Build history of the part. All positions in model axes, mm. Face numbers are marked on the shaded views. A direction names the side the tool comes from. Give positions to 0.01 mm unless a question says otherwise; leave off trailing zeros. Loops run counter-clockwise (first coordinate to the right, second up) from the corner with the lowest first, then second, coordinate; pieces in that order, holes last. Notation, with made-up numbers: (5, 16) -> (18, 16) arc R24 cw to (18, 39) -> close; hole circle Ø5 at (-36, 16.25). An arc over 180 degrees is marked (long way). Answer as a JSON object with one key per item and string values. Group by question number.
Q1. Two-plate mould, pull along X, no slides. Class the marked faces 3, 4 and 5: pulls with the +X half, pulls with the -X half, needs draft (parallel to the pull), parting line crosses it, or undercut.
Q2. Band-saw the part on B-B, the plane y = 1. Write the cut outline in (x, z), plus the area to 3 significant figures.
Q3. Drop flat-ended pins along their axis: pin 1 (1 mm diameter, centred on x = -6.5, y = 8, fed in from -Z); pin 2 (5 mm diameter, centred on x = -2.5, z = 5.5, fed in from +Y); pin 3 (3 mm diameter, centred on x = 5.5, z = 1, fed in from +Y). Give the stop position or say it passes through.
Q4. Band-saw the part on A-A, the plane z = 8. Write the cut outline in (x, y).
Q5. Wall check: probe 1 along X at (y, z) = (2.3, 0); probe 2 along Z at (x, y) = (0, 1.2). Give the ranges that are in metal, low to high. Write a range as from..to.
Q6. Tool access for the marked faces 1 and 2: list every direction of +Z, -Z, +X, -X, +Y, -Y with a clear straight run to the whole face (end or side of a thin tool).
from build123d import *

# Parameters (mm, degrees)
SKETCH4_R          = 4.7752
CUT_EXTRUDE1_DEPTH = 12.446
FILLET2_R          = 5.08


with BuildPart() as part:
    # Sketch3 → Revolve3 (revolve)
    with BuildSketch(Plane.XY):
        Polygon((7.1628, 1.8288), (7.1628, 5.1054), (0, 5.1054), (0, 0), (9.398, 0), (9.398, 1.8288), align=None)
        with BuildLine():
            ThreePointArc((0, 5.1054), (5.231120596, 6.316339666), (9.398, 9.7028))
            Line((9.398, 9.7028), (9.398, 5.1054))
            Line((9.398, 5.1054), (7.1628, 5.1054))
            Line((7.1628, 5.1054), (0, 5.1054))
        make_face()
    revolve(axis=Axis((0, 0, 0), (0, 1, 0)))

    # Sketch4 → Cut-Extrude1 (cut)
    with BuildSketch(Plane.XZ):
        Circle(SKETCH4_R)
    extrude(amount=-CUT_EXTRUDE1_DEPTH, mode=Mode.SUBTRACT)

    # Fillet2
    fillet2_edges = [part.edges().sort_by_distance(p)[0] for p in [
        (-4.7752, 6.105113597, 2e-09),
    ]]
    fillet(fillet2_edges, radius=FILLET2_R)


solid = part.part
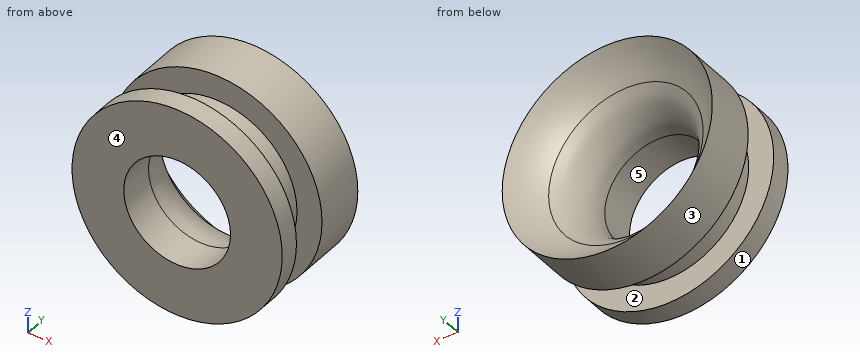
Worked answers:
{
 "1": {"face 3": "parting line crosses it", "face 4": "needs draft", "face 5": "undercut"},
 "2": {"outline": "circle Ø18.8 at (0, 0); hole circle Ø9.55 at (0, 0)", "area": "206 mm2"},
 "3": {"pin 1": "z = -7.23", "pin 2": "y = 8.72", "pin 3": "y = 7.45"},
 "4": {"outline": "(-4.93, 0) -> (4.93, 0) -> (4.93, 1.83) -> (-4.93, 1.83) -> close; (-4.93, 5.11) -> (4.93, 5.11) -> (4.93, 9.7) arc R8.82 cw to (-4.93, 9.7) -> close"},
 "5": {"probe 1": "-7.16..-4.78, 4.78..7.16", "probe 2": "-9.4..-4.78, 4.78..9.4"},
 "6": {"face 1": "+Y, -Y", "face 2": "none"}
}
